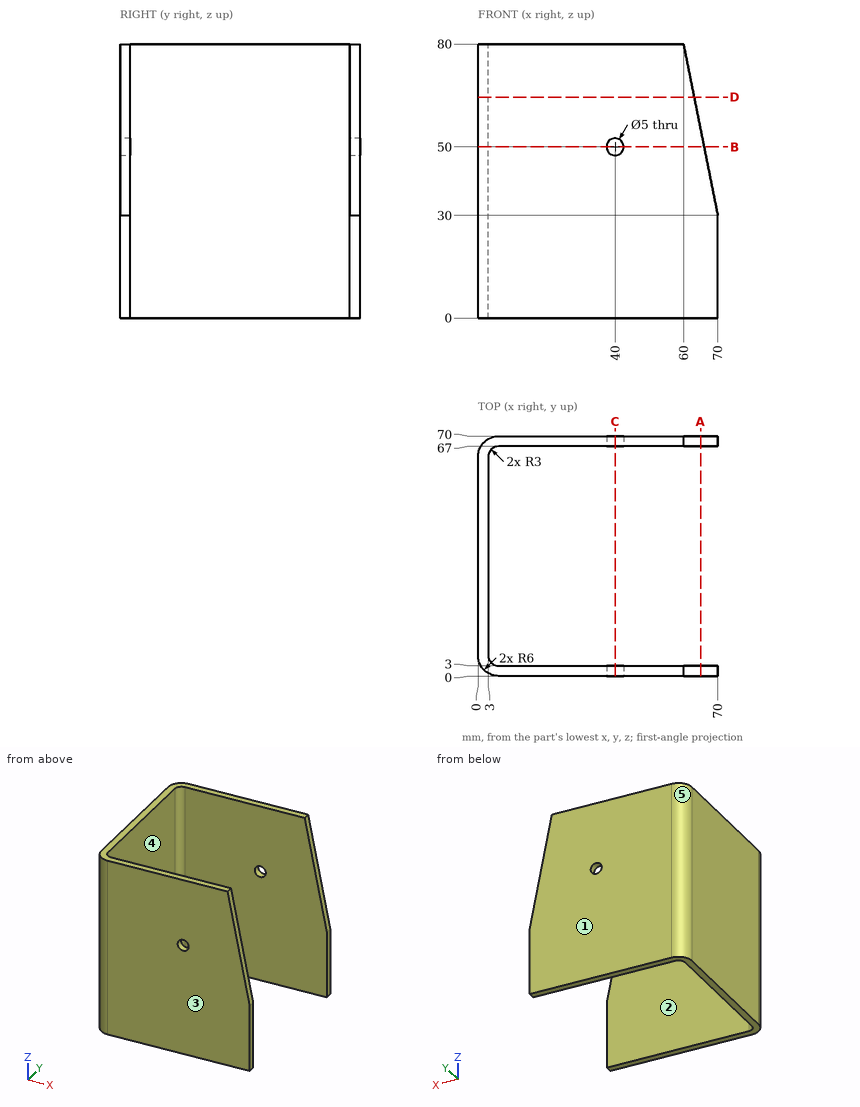
Answer from the drawing. Dimensions are ordinates in mm from the lowest x, y and z of the part. A direction names the side the tool comes from. Coordinates: 2 decimals unless noted, no trailing zeros. Write each loop counter-clockwise with the first axis right and the second up, starting at its lowest first coordinate (ties: lowest second). Pieces come first, ordered by that corner, then holes. Notation, with made-up numbers: M 72.5,42.5 L 78.5,42.5 A9 ccw 78.5,48.5 Z; hole C -30,51.5 d10. An arc over 180 degrees is marked long. Use one line per item in the form item = value. Start each with the question number.
1. The mould has two halves that part along Y. Classify the marked faces 1, 2 and 3: released by +Y, released by -Y, zero draft, split by the parting line, or undercut.
2. The part is cut by section B-B (z = 50). Give the vertices of the cut face in (x, y), plus the area to 3 significant figures.
3. Straight lines are drawn through the part: probe 1 along Y at (x, z) = (9, 35); probe 2 along X at (y, z) = (47, 56); probe 3 along X at (y, z) = (68.15, 50). For each, find the intervals that lie inside material, in ascending order. Write a range as from..to.
4. A tool of negligible diameter and unlimited length cuts with its end or side. For the marked faces 4 and 5, from which of +Z, -Z, +X, -X, +Y, -Y can it reach the whole face along a straight path? Write none if from no direction.
5. This flat-tipped pin is pushed along its axis until it touches: P1, Ø8, axis at y = 24, z = 65.5, coming from the +X side. Where does it stop, or does it pass through?
6. The part is cut by section A-A (x = 65). Give the vertices of the cut face in (y, z).
7. The part is cut by section C-C (x = 40). Give the vertices of the cut face in (y, z), plus the area to 3 significant figures.
8. The part is cut by section D-D (z = 64.5). Give the vertices of the cut face in (x, y).
Evaluation:
q1.face_1 = released by +Y
q1.face_2 = undercut
q1.face_3 = released by -Y
q2.outline = M 0,6 A6 ccw 6,0 L 37.5,0 L 37.5,3 L 6,3 A3 cw 3,6 L 3,64 A3 cw 6,67 L 37.5,67 L 37.5,70 L 6,70 A6 ccw 0,64 Z; M 42.5,0 L 66,0 L 66,3 L 42.5,3 Z; M 42.5,67 L 66,67 L 66,70 L 42.5,70 Z
q2.area = 546 mm^2
q3.probe_1 = 0..3, 67..70
q3.probe_2 = 0..3
q3.probe_3 = 1.67..37.5, 42.5..66
q4.face_4 = +Z, -Z, +X
q4.face_5 = +Z, -Z, -X, +Y
q5.P1 = 3
q6.outline = M 0,0 L 3,0 L 3,55 L 0,55 Z; M 67,0 L 70,0 L 70,55 L 67,55 Z
q7.outline = M 0,0 L 3,0 L 3,47.5 L 0,47.5 Z; M 0,52.5 L 3,52.5 L 3,80 L 0,80 Z; M 67,0 L 70,0 L 70,47.5 L 67,47.5 Z; M 67,52.5 L 70,52.5 L 70,80 L 67,80 Z
q7.area = 450 mm^2
q8.outline = M 0,6 A6 ccw 6,0 L 63.1,0 L 63.1,3 L 6,3 A3 cw 3,6 L 3,64 A3 cw 6,67 L 63.1,67 L 63.1,70 L 6,70 A6 ccw 0,64 Z
